```python
from build123d import *

# Parameters (mm, degrees)
F0_R      = 4.875
F1_DEPTH  = 7
F3_DEPTH  = 5
F4_R      = 1.25
F5_DEPTH  = 5
F6_W      = 0.9999981817
F6_H      = 0.5
F6_W_2    = 1
F6_H_2    = 0.75
F6_W_3    = 0.65
F6_H_3    = 4.3095893331
F8_DEPTH  = 1
F10_R     = 1.375
F10_R_2   = 1.25
F11_DEPTH = 0.15
F13_R     = 1.375
F13_R_2   = 1.25
F14_DEPTH = 0.15


with BuildPart() as f1:
    # F0 (on Top) → F1 (new body)
    with BuildSketch(Plane.XY):
        Circle(F0_R)
    extrude(amount=F1_DEPTH)

    # F2 (on Front) → F3 (cut, symmetric)
    with BuildSketch(Plane.XZ):
        with BuildLine():
            Line((-4, 0), (-4, 3.3174325915))
            ThreePointArc((-4, 3.3174325915), (-4.2928932188, 4.0245393727), (-5, 4.3174325915))
            Line((-5, 4.3174325915), (-5, 0))
            Line((-5, 0), (-4, 0))
        make_face()
        with BuildLine():
            ThreePointArc((5, 4.3174325915), (4.2928932188, 4.0245393727), (4, 3.3174325915))
            Line((4, 3.3174325915), (4, 0))
            Line((4, 0), (5, 0))
            Line((5, 0), (5, 4.3174325915))
        make_face()
    extrude(amount=F3_DEPTH, both=True, mode=Mode.SUBTRACT)

    # F4 (on Right) → F5 (cut, symmetric)
    with BuildSketch(Plane.YZ):
        with Locations((0, 1.9518149326)):
            Circle(F4_R)
    extrude(amount=F5_DEPTH, both=True, mode=Mode.SUBTRACT)

    # F6 (on Front) → F7 (revolve, cut)
    with BuildSketch(Plane.XZ):
        with Locations((4.875, 6.5)):
            Rectangle(F6_W, F6_H)
        with Locations((4.875, 5.75)):
            Rectangle(F6_W_2, F6_H)
        with Locations((4.875, 4.875)):
            Rectangle(F6_W_2, F6_H_2)
        with Locations((5.05, 2.1547946666)):
            Rectangle(F6_W_3, F6_H_3)
    revolve(axis=Axis((0, 0, 3.6421683617), (0, 0, 1)), mode=Mode.SUBTRACT)

    # F8 (add): a face of the model
    f8_faces = [f1.faces().sort_by_distance(p)[0] for p in [
        (0, 0, 7),
    ]]
    extrude(f8_faces, amount=F8_DEPTH)

    # F10 (on offset) → F11 (cut)
    with BuildSketch(Plane.YZ.offset(3.75)):
        with Locations((0, 1.9518149326)):
            Circle(F10_R)
        with Locations((0, 1.9518149326)):
            Circle(F10_R_2, mode=Mode.SUBTRACT)
    extrude(amount=-F11_DEPTH, mode=Mode.SUBTRACT)

    # F13 (on offset) → F14 (cut)
    with BuildSketch(Plane(origin=(-3.75, 0, 0), x_dir=(0, -1, 0), z_dir=(-1, 0, 0))):
        with Locations((0, 1.9518149326)):
            Circle(F13_R)
        with Locations((0, 1.9518149326)):
            Circle(F13_R_2, mode=Mode.SUBTRACT)
    extrude(amount=-F14_DEPTH, mode=Mode.SUBTRACT)


solid = f1.part
```
Verification items for the finished model (mm, model axes). A direction names the side the tool comes from. Give positions to 0.01 mm unless a question says otherwise; leave off trailing zeros. Order: outer loops, then holes, each group sorted by start corner. A loop starts at its lowest first (then second) coordinate and runs counter-clockwise, first axis right, second up. Notation, with made-up numbers: M -28,-3 L 10,-3 A34 ccw 10,29 Z; hole C 89,83 d4. An arc over 180 degrees is marked long. Return JSON: item names as keys, results as strings. Group by question number.
1) Scan lines: line 1 (Z direction, x = -0.75, y = 4.75); line 2 (Z direction, x = -2.5, y = -3.75); line 3 (Z direction, x = -1, y = 0). Record each from-to range of solid material in increasing order.
2) Access from +Z, -Z, +X, -X, +Y, -Y to the whole of each face (thin tool, end or side, straight path). Record for faces 1 (the face through (-3.472, -2.662, 5.754)), 2 (the face through (0, 0, 0)), 3 (the face through (4, -0.6, 0.6)).
3) Section check D-D on z = 1.5. Record the cut outline in (x, y) (3 decimals), and give its area (3 significant figures).
4) Section check A-A on z = 2.75. Record the cut outline in (x, y) (3 decimals).
5) Go/stop test with flat-tipped pins: pin 1 Ø3 at (y, z) = (0, 1.95) entering from +X; pin 2 Ø1.5 at (y, z) = (2.5, 5.5) entering from +X; pin 3 Ø3 at (y, z) = (-3, 5.5) entering from +X. Record where each tip stops, or that it passes through.
Answer block:
{
 "1": {"line 1": "z = 4.31 to 4.5, 5.25 to 5.5, 6 to 6.25, 6.75 to 8", "line 2": "z = 0 to 4.5, 5.25 to 5.5, 6 to 6.25, 6.75 to 8", "line 3": "z = 0 to 0.7, 3.2 to 8"},
 "2": {"face 1": "none", "face 2": "-Z, +X, -X, +Y, -Y", "face 3": "-Z, +X, +Y, -Y"},
 "3": {"outline": "M -4,-2.515 A4.725 ccw 4,-2.515 L 4,-1.165 L 3.75,-1.165 L 3.75,-1.299 L 3.6,-1.299 L 3.6,-1.165 L -3.6,-1.165 L -3.6,-1.299 L -3.75,-1.299 L -3.75,-1.165 L -4,-1.165 Z; M -4,1.165 L -3.75,1.165 L -3.75,1.299 L -3.6,1.299 L -3.6,1.165 L 3.6,1.165 L 3.6,1.299 L 3.75,1.299 L 3.75,1.165 L 4,1.165 L 4,2.515 A4.725 ccw -4,2.515 Z", "area": "46.5 mm^2"},
 "4": {"outline": "M -4,-2.515 A4.725 ccw 4,-2.515 L 4,-0.962 L 3.75,-0.962 L 3.75,-1.12 L 3.6,-1.12 L 3.6,-0.962 L -3.6,-0.962 L -3.6,-1.12 L -3.75,-1.12 L -3.75,-0.962 L -4,-0.962 Z; M -4,0.962 L -3.75,0.962 L -3.75,1.12 L -3.6,1.12 L -3.6,0.962 L 3.6,0.962 L 3.6,1.12 L 3.75,1.12 L 3.75,0.962 L 4,0.962 L 4,2.515 A4.725 ccw -4,2.515 Z"},
 "5": {"pin 1": "stops at x = 4.01", "pin 2": "stops at x = 4.55", "pin 3": "stops at x = 4.64"}
}
